Build history of the part. All positions in model axes, mm. Round coordinates to 2 decimals unless told otherwise and drop trailing zeros. Write each loop counter-clockwise with the first axis right and the second up, starting at its lowest first coordinate (ties: lowest second). Pieces come first, ordered by that corner, then holes. Notation, with made-up numbers: (-31, -30.5) - (4, -30.5) arc R18 cw to (4, -19.5) - close; hole circle Ø9 at (-14.75, 7.25). An arc over 180 degrees is marked (long way). Answer as a JSON object with one key per item and string values. Group by question number.
Item 1: Slice it at C-C, the plane z = 0.9. List the corners of the cut face in (x, y) (1 decimal).
Item 2: Slice it at A-A, the plane y = 10.5. List the corners of the cut face in (x, z).
Item 3: Probe line 1 (Y direction, x = 28.5, z = 1); line 2 (X direction, y = -10.75, z = 0.55); line 3 (Y direction, x = 8.5, z = 1). List the from-to ranges inside material, lowest first. Write a range as from..to.
Item 4: Flat gauge pin, fed straight in: pin 1 (1 mm diameter, centred on x = 7, y = 0.5, fed in from -Z). Where does the tip first touch, or does it go through?
Item 5: Slice it at B-B, the plane x = 17. List the corners of the cut face in (y, z).
Item 6: Slice it at D-D, the plane y = 1. List the corners of the cut face in (x, z).
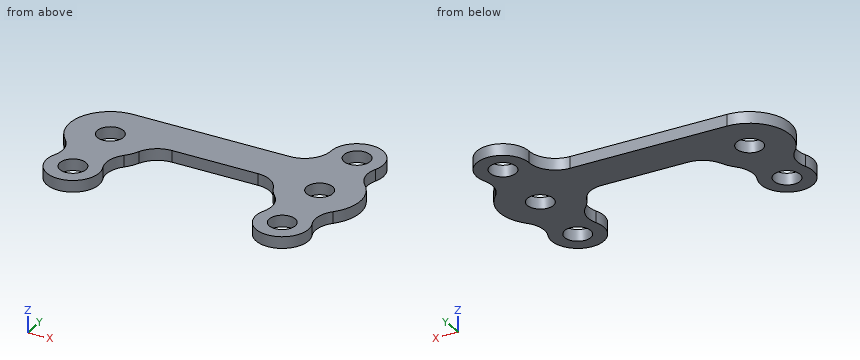
from build123d import *

# Parameters (mm, degrees)
SKETCH1_R           = 1.7859375
BOSS_EXTRUDE1_DEPTH = 1.5875
FILLET1_R           = 3.571875


with BuildPart() as part:
    # Sketch1 → Boss-Extrude1 (new body)
    with BuildSketch(Plane.XY):
        with BuildLine():
            ThreePointArc((4.001636181, -3.854714248), (5.152960561, -2.078199104), (5.55625, 0))
            Line((5.55625, 0), (23.01875, 0))
            ThreePointArc((23.01875, 0), (23.422039397, -2.078199001), (24.573363664, -3.854714088))
            ThreePointArc((24.573363664, -3.854714088), (25.513553345, -5.68510334), (25.287941571, -7.730434799))
            ThreePointArc((25.287941571, -7.730434799), (28.575000018, -12.7), (31.862058415, -7.730434766))
            ThreePointArc((31.862058415, -7.730434766), (31.636446643, -5.685103406), (32.576636217, -3.854714211))
            ThreePointArc((32.576636217, -3.854714211), (34.13125, -2e-08), (32.576636245, 3.854714182))
            ThreePointArc((32.576636245, 3.854714182), (31.636446652, 5.685103357), (31.862058392, 7.730434711))
            ThreePointArc((31.862058392, 7.730434711), (29.288207306, 12.628071622), (25.003125, 9.128125))
            ThreePointArc((25.003125, 9.128125), (23.956947034, 6.602427966), (21.43125, 5.55625))
            Line((21.43125, 5.55625), (0, 5.55625))
            ThreePointArc((0, 5.55625), (-5.113202033, 2.174184683), (-4.00163619, -3.85471424))
            ThreePointArc((-4.00163619, -3.85471424), (-3.061446646, -5.685103393), (-3.287058389, -7.730434703))
            ThreePointArc((-3.287058389, -7.730434703), (1.4e-08, -12.7), (3.287058378, -7.730434678))
            ThreePointArc((3.287058378, -7.730434678), (3.061446647, -5.685103385), (4.001636181, -3.854714248))
        make_face()
        Circle(SKETCH1_R, mode=Mode.SUBTRACT)
        with Locations((28.575, 0)):
            Circle(SKETCH1_R, mode=Mode.SUBTRACT)
        with Locations((0, -9.128125)):
            Circle(SKETCH1_R, mode=Mode.SUBTRACT)
        with Locations((28.575, -9.128125)):
            Circle(SKETCH1_R, mode=Mode.SUBTRACT)
        with Locations((28.575, 9.128125)):
            Circle(SKETCH1_R, mode=Mode.SUBTRACT)
    extrude(amount=BOSS_EXTRUDE1_DEPTH)

    # Fillet1
    fillet1_edges = [part.edges().sort_by_distance(p)[0] for p in [
        (23.01875, 0, 0.79375),
        (5.55625, 0, 0.79375),
    ]]
    fillet(fillet1_edges, radius=FILLET1_R)


solid = part.part
Geometry says:
{
 "1": {"outline": "(-4, -3.9) arc R3.6 cw to (-3.3, -7.7) arc R3.6 ccw (long way) to (3.3, -7.7) arc R3.6 cw to (4, -3.9) arc R5.6 ccw to (5.1, -2.2) arc R3.6 cw to (8.4, 0) - (20.2, 0) arc R3.6 cw to (23.5, -2.2) arc R5.6 ccw to (24.6, -3.9) arc R3.6 cw to (25.3, -7.7) arc R3.6 ccw (long way) to (31.9, -7.7) arc R3.6 cw to (32.6, -3.9) arc R5.6 ccw to (32.6, 3.9) arc R3.6 cw to (31.9, 7.7) arc R3.6 ccw (long way) to (25, 9.1) arc R3.6 cw to (21.4, 5.6) - (0, 5.6) arc R5.6 ccw to start; hole circle Ø3.6 at (0, -9.1); hole circle Ø3.6 at (0, 0); hole circle Ø3.6 at (28.6, -9.1); hole circle Ø3.6 at (28.6, 0); hole circle Ø3.6 at (28.6, 9.1)"},
 "2": {"outline": "(25.28, 0) - (27.43, 0) - (27.43, 1.59) - (25.28, 1.59) - close; (29.72, 0) - (31.87, 0) - (31.87, 1.59) - (29.72, 1.59) - close"},
 "3": {"line 1": "y = -12.7..-10.91, -7.34..-1.78, 1.78..7.34, 10.91..12.7", "line 2": "x = -3.18..-0.75, 0.75..3.18, 25.39..27.83, 29.32..31.76", "line 3": "y = 0..5.56"},
 "4": {"pin 1": "stops at z = 0"},
 "5": {"outline": "(0, 0) - (5.56, 0) - (5.56, 1.59) - (0, 1.59) - close"},
 "6": {"outline": "(-5.47, 0) - (-1.48, 0) - (-1.48, 1.59) - (-5.47, 1.59) - close; (1.48, 0) - (27.1, 0) - (27.1, 1.59) - (1.48, 1.59) - close; (30.05, 0) - (34.04, 0) - (34.04, 1.59) - (30.05, 1.59) - close"}
}
